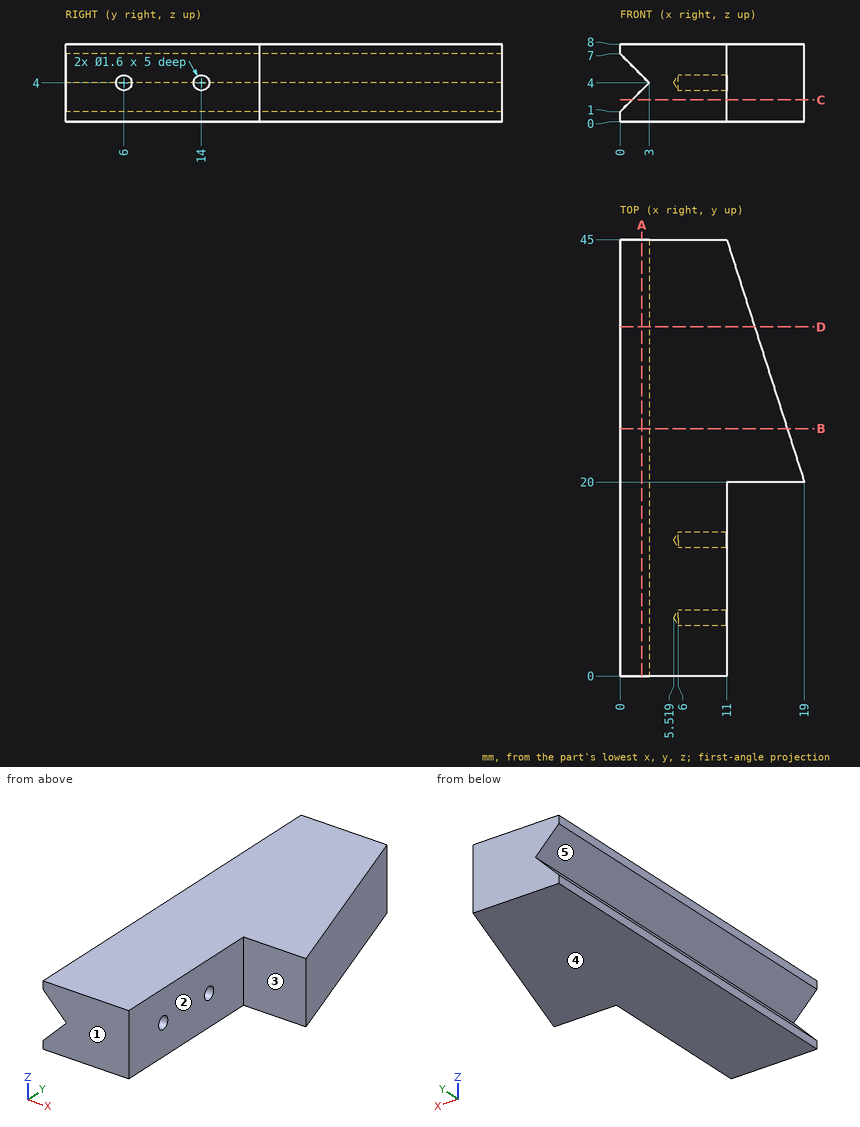
Input: dimensioned drawing with shaded views. Units: mm. Origin: part minimum x, y, z. A direction names the side the tool comes from. Give positions to 0.01 mm unless a question says otherwise; leave off trailing zeros. Write each loop counter-clockwise with the first axis right and the second up, starting at its lowest first coordinate (ties: lowest second). Pieces come first, ordered by that corner, then holes. Notation, with made-up numbers: (-31, 73.25) -> (-16, 73.25) arc R26 cw to (-16, 108.25) -> close; hole circle Ø4 at (70, 25). An arc over 180 degrees is marked (long way). Return JSON: item names as keys, results as strings. Group by question number.
1. Section B-B, the plane y = 25.5. Output: boundary loops of the cut face in (x, z).
2. Section A-A, the plane x = 2.25. Output: boundary loops of the cut face in (y, z).
3. Section D-D, the plane y = 36. Output: boundary loops of the cut face in (x, z), then the cut area to 3 significant figures.
4. Material intervals for line 1 (Y direction, x = 9.1, z = 4); line 2 (X direction, y = 3.5, z = 7.25); line 3 (X direction, y = 8, z = 6), sorted ascending. Write a range as from..to.
5. Access query for the marked faces 1 and 2. Directions: +Z, -Z, +X, -X, +Y, -Y. A direction counts if a zero-diameter tool reaches every point of the face in a straight line with its end or side. Return the directions, or none.
6. Section C-C, the plane z = 2.25. Output: boundary loops of the cut face in (x, y), then the cut area to 3 significant figures.
7. Pin query (flat end, axial travel): pin 1 Ø1.5 at (x, z) = (13, 7) entering from -Y; pin 2 Ø2.5 at (y, z) = (14, 4) entering from +X; pin 3 Ø1.3 at (y, z) = (6, 4) entering from +X. Return the tip coordinate at first contact, or that it passes through.
8. Mould query, pull axis Z, two halves, no side actions, for the marked faces 3, 4 and 5. Classes: +Z half, -Z half, draft (parallel to the pull), parting line (faces both ways), or undercut.
Determined:
{
 "1": {"outline": "(0, 0) -> (17.24, 0) -> (17.24, 8) -> (0, 8) -> (0, 7) -> (3, 4) -> (0, 1) -> close"},
 "2": {"outline": "(0, 0) -> (45, 0) -> (45, 3.25) -> (0, 3.25) -> close; (0, 4.75) -> (45, 4.75) -> (45, 8) -> (0, 8) -> close"},
 "3": {"outline": "(0, 0) -> (13.88, 0) -> (13.88, 8) -> (0, 8) -> (0, 7) -> (3, 4) -> (0, 1) -> close", "area": "102 mm2"},
 "4": {"line 1": "y = 0..5.2, 6.8..13.2, 14.8..45", "line 2": "x = 0..11", "line 3": "x = 1..11"},
 "5": {"face 1": "+Z, -Z, +X, -X, -Y", "face 2": "+Z, -Z, +X, -Y"},
 "6": {"outline": "(1.25, 0) -> (11, 0) -> (11, 20) -> (19, 20) -> (11, 45) -> (1.25, 45) -> close", "area": "539 mm2"},
 "7": {"pin 1": "stops at y = 20", "pin 2": "stops at x = 11", "pin 3": "stops at x = 5.91"},
 "8": {"face 3": "draft", "face 4": "-Z half", "face 5": "undercut"}
}
